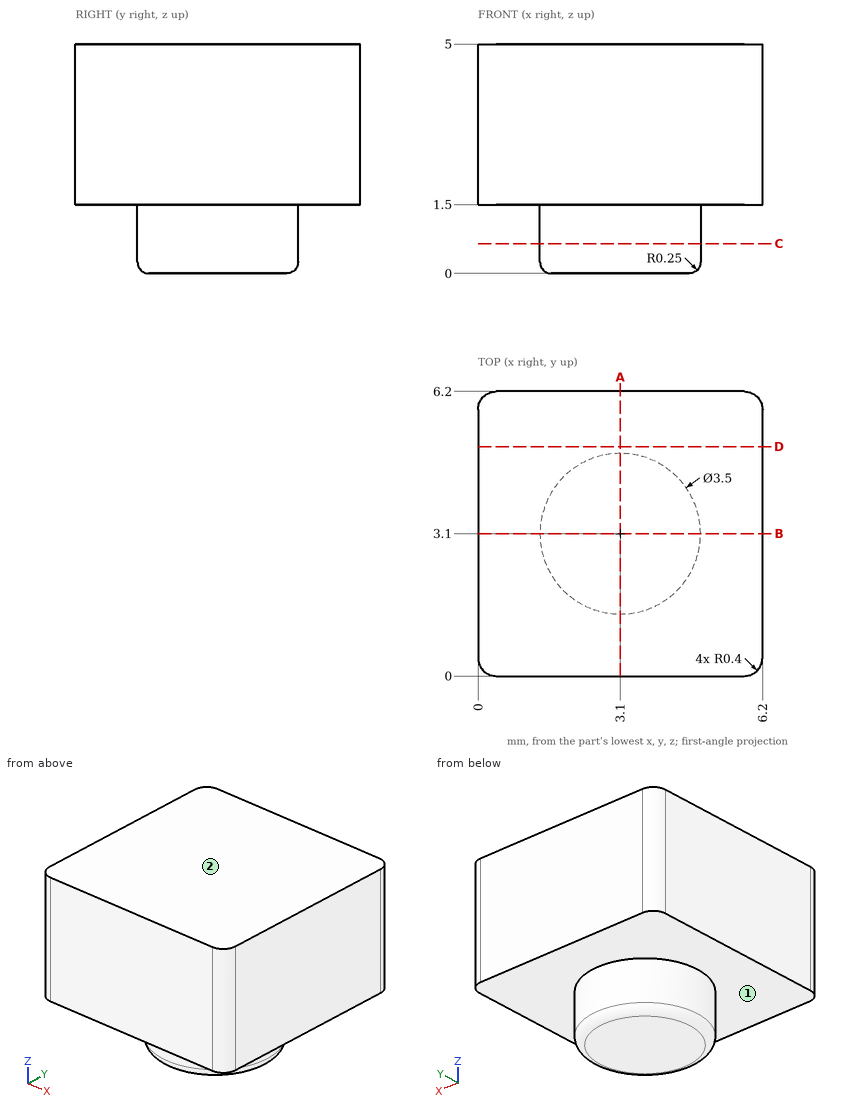
Geometry check sheet. Reference: drawing and pictorial views, mm from the part's lowest x, y, z. A direction names the side the tool comes from. Round coordinates to 2 decimals unless told otherwise and drop trailing zeros. Loops run counter-clockwise (first coordinate to the right, second up) from the corner with the lowest first, then second, coordinate; pieces in that order, holes last. Notation, with made-up numbers: (38, -40) - (65, -40) arc R17 ccw to (65, -9) - close; hole circle Ø5 at (-7, 55.5). An arc over 180 degrees is marked (long way). Write item = value, one per line. Start each with the question number.
Q1. Section check D-D (y = 5). Record the boundary of the cut face in (x, z), plus the area to 3 significant figures.
Q2. Access from +Z, -Z, +X, -X, +Y, -Y to the whole of each face (thin tool, end or side, straight path). Record for the marked faces 1 and 2.
Q3. Thickness scan on L1, parallel to Z at x = 0.75, y = 4.5; L2, parallel to X at y = 3, z = 0.5; L3, parallel to Z at x = 3, y = 1.5. Record the ranges inside material, lowest first.
Q4. Section check C-C (z = 0.65). Record the boundary of the cut face in (x, y).
Q5. Section check A-A (x = 3.1). Record the boundary of the cut face in (y, z), plus the area to 3 significant figures.
Derived:
q1.outline = (0, 1.5) - (6.2, 1.5) - (6.2, 5) - (0, 5) - close
q1.area = 21.7 mm^2
q2.face_1 = -Z
q2.face_2 = +Z, +X, -X, +Y, -Y
q3.L1 = 1.5 to 5
q3.L2 = 1.35 to 4.85
q3.L3 = 0.02 to 5
q4.outline = circle Ø3.5 at (3.1, 3.1)
q5.outline = (0, 1.5) - (1.35, 1.5) - (1.35, 0.25) arc R0.25 ccw to (1.6, 0) - (4.6, 0) arc R0.25 ccw to (4.85, 0.25) - (4.85, 1.5) - (6.2, 1.5) - (6.2, 5) - (0, 5) - close
q5.area = 26.9 mm^2
